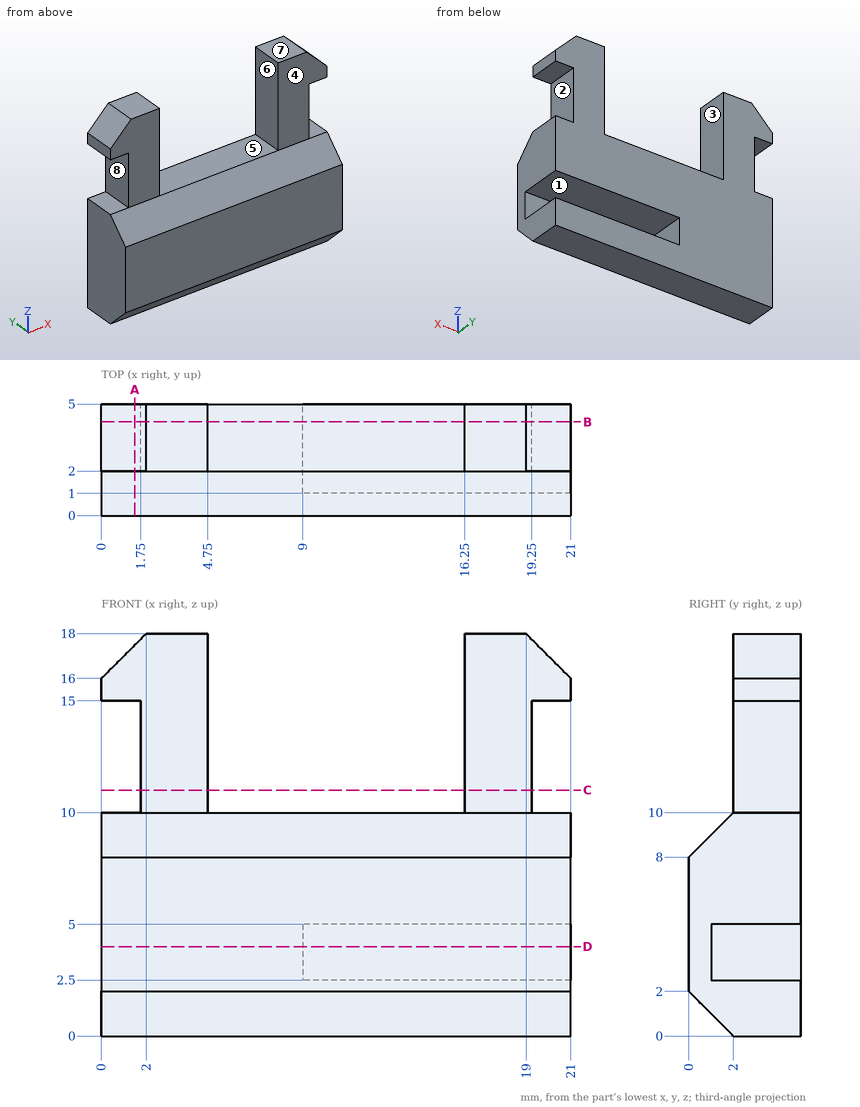
Verification items for this drawing (mm, ordinates from the low corner). A direction names the side the tool comes from. Round coordinates to 2 decimals unless told otherwise and drop trailing zeros. Order: outer loops, then holes, each group sorted by start corner. A loop starts at its lowest first (then second) coordinate and runs counter-clockwise, first axis right, second up. Notation, with made-up numbers: (14, 14) - (65, 14) arc R23 cw to (65, 34) - close; hole circle Ø2 at (-12, 28). An arc over 180 degrees is marked (long way). Use CSV: the item, a comma, the result in double quotes. Start each with the question number.
1) Access from +Z, -Z, +X, -X, +Y, -Y to the whole of each face (thin tool, end or side, straight path). Record for the marked faces 1, 2, 3 and 4.
2) Section check C-C, the plane z = 11. Record the cut outline in (x, y).
3) Section check A-A, the plane x = 1.5. Record the cut outline in (y, z), plus the area to 3 significant figures.
4) Section check B-B, the plane y = 4.2. Record the cut outline in (x, z), plus the area to 4 significant figures.
5) Thickness scan on L1, parallel to Z at x = 11.75, y = 2.35; L2, parallel to X at y = 2.2, z = 11.75; L3, parallel to Z at x = 5, y = 3.8. Record the ranges inside material, lowest first.
6) Mould release check, pull along Z, two halves, no side actions. Record for the marked faces 5, 6, 7 and 8: +Z half, -Z half, draft (parallel to the pull), parting line (faces both ways), or undercut.
7) Go/stop test with flat-tipped pins: P1, Ø5, axis at x = 19, z = 16, coming from the -Y side; P2, Ø0.9, axis at x = 12, y = 3.5, coming from the +Z side; P3, Ø0.9, axis at y = 3, z = 14.5, coming from the -X side. Record where each tip stops, or that it passes through.
8) Section check D-D, the plane z = 4. Record the cut outline in (x, y), plus the area to 3 significant figures.
Answers:
1,face 1,"+X, +Y"
1,face 2,"+X, +Y, -Y"
1,face 3,"+Z, +Y, -Y"
1,face 4,"+Z, +X, -X, -Y"
2,outline,"(1.75, 2) - (4.75, 2) - (4.75, 5) - (1.75, 5) - close; (16.25, 2) - (19.25, 2) - (19.25, 5) - (16.25, 5) - close"
3,outline,"(0, 2) - (2, 0) - (5, 0) - (5, 10) - (2, 10) - (0, 8) - close; (2, 15) - (5, 15) - (5, 17.5) - (2, 17.5) - close"
3,area,"53.5 mm²"
4,outline,"(0, 0) - (21, 0) - (21, 2.5) - (9, 2.5) - (9, 5) - (21, 5) - (21, 10) - (19.25, 10) - (19.25, 15) - (21, 15) - (21, 16) - (19, 18) - (16.25, 18) - (16.25, 10) - (4.75, 10) - (4.75, 18) - (2, 18) - (0, 16) - (0, 15) - (1.75, 15) - (1.75, 10) - (0, 10) - close"
4,area,"234.5 mm²"
5,L1,"z = 0 to 2.5, 5 to 10"
5,L2,"x = 1.75 to 4.75, 16.25 to 19.25"
5,L3,"z = 0 to 10"
6,face 5,"+Z half"
6,face 6,"draft"
6,face 7,"+Z half"
6,face 8,"undercut"
7,P1,"stops at y = 2"
7,P2,"stops at z = 10"
7,P3,"stops at x = 1.75"
8,outline,"(0, 0) - (21, 0) - (21, 1) - (9, 1) - (9, 5) - (0, 5) - close"
8,area,"57.0 mm²"
